Here's how the part is built. I have some questions about the finished solid (model axes, mm). A direction names the side the tool comes from. Round coordinates to 2 decimals unless told otherwise and drop trailing zeros. Write item = value, one per line. Start each with the question number.
(1) On a 3-axis mill with a long thin cutter (end or side, diameter ignored), from which of +Z, -Z, +X, -X, +Y, -Y can I reach the whole of each face in a straight line? I mean faces 4 (the cylindrical face through (95.78, -4.1, 144.76)), 5 (the cylindrical face through (127.856, -12.905, 148.568)), 6 (the flat face through (138.989, 0, 132)). Say none if no direction works.
(2) If we mould it in two halves opening along Z, with no side actions, what happens to faces 1 (the flat face through (70.307, -14, 132)), 2 (the cylindrical face through (-221.722, -170.011, -6.439)), 3 (the flat face through (0, 0, 158.217))? For each: released by +Z, released by -Z, zero draft, split by the parting line, or undercut.
(3) Will these pins go through, and if not, where does the flat tip stop? pin 1 Ø12 at (x, y) = (145, 214.5) entering from +Z; pin 2 Ø21 at (y, z) = (7.5, 141) entering from -X; pin 3 Ø1.5 at (x, z) = (123, 2) entering from +Y.
(4) I need wall thicknesses on line 1 along Z through (x, y) = (205, 138.5); line 2 along Z through (x, y) = (124.5, 5); line 3 along Y through (x, z) = (32.5, 5.5). Which ranges of each line are inside material? Lowest first, please.
```python
from build123d import *

# Parameters (mm, degrees)
EXTRUSION1_DEPTH      = 25.4
EXTRUSION1_DEPTH_BACK = 38.1
SKETCH1_R             = 279.4
FILLET1_R             = 25.4
SKETCH2_R             = 48.9585
EXTRUSION2_DEPTH      = 37.211
SKETCH3_R             = 14.9225
EXTRUSION3_DEPTH      = 95.6056
SKETCH4_R             = 13.6525
EXTRUSION4_DEPTH      = 133.8072
EXTRUSION5_START      = -80.4672
SKETCH5_R             = 21.209
SKETCH5_R_2           = 13.6525
EXTRUSION5_DEPTH      = 80.4672
EXTRUSION6_START      = -63.5
SKETCH6_R             = 21.209
EXTRUSION6_DEPTH      = 63.5
SKETCH7_R             = 13.6525
EXTRUSION7_DEPTH      = 51.6636
SKETCH8_R             = 21.209
EXTRUSION8_DEPTH      = 17.018
FILLET2_R             = 5.08


with BuildPart() as part:
    # Sketch1 → Extrusion1 (new, two sides: drawn at the far end of the back side and taken through both)
    with BuildSketch(Plane.XY.offset(-EXTRUSION1_DEPTH_BACK)):
        Circle(SKETCH1_R)
    extrude(amount=EXTRUSION1_DEPTH + EXTRUSION1_DEPTH_BACK)

    # Fillet1
    fillet1_edges = [part.edges().sort_by_distance(p)[0] for p in [
        (-279.4, 0, -38.1),
        (-279.4, 0, 25.4),
    ]]
    fillet(fillet1_edges, radius=FILLET1_R - 0.0001)  # a hair under: the kernel refuses the full size

    # Sketch2 → Extrusion2 (add)
    with BuildSketch(Plane.XY.offset(25.4)):
        with Locations(Location((0, 0, 0), (0, 0, 180))):
            Circle(SKETCH2_R)
    extrude(amount=EXTRUSION2_DEPTH)

    # Sketch3 → Extrusion3 (add)
    with BuildSketch(Plane.XY.offset(62.611)):
        Circle(SKETCH3_R)
    extrude(amount=EXTRUSION3_DEPTH)

    # Sketch4 → Extrusion4 (add)
    with BuildSketch(Plane.YZ):
        with Locations(Location((0, 131.7371, 0), (0, 0, 270))):
            Circle(SKETCH4_R)
    extrude(amount=EXTRUSION4_DEPTH)

    # Sketch5 → Extrusion5 (add)
    with BuildSketch(Plane(origin=(133.8072, 0, 0), x_dir=(0, 0, -1), z_dir=(1, 0, 0)).offset(EXTRUSION5_START)):
        with Locations((-131.7371, 0)):
            Circle(SKETCH5_R)
        with Locations(Location((-131.7371, 0, 0), (0, 0, 180))):
            Circle(SKETCH5_R_2, mode=Mode.SUBTRACT)
    extrude(amount=EXTRUSION5_DEPTH)

    # Sketch6 → Extrusion6 (cut)
    with BuildSketch(Plane(origin=(133.8072, 0, 0), x_dir=(0, 0, -1), z_dir=(1, 0, 0)).offset(EXTRUSION6_START)):
        with Locations((-131.7371, 0)):
            Circle(SKETCH6_R)
    extrude(amount=EXTRUSION6_DEPTH, mode=Mode.SUBTRACT)

    # Sketch7 → Extrusion7 (add)
    with BuildSketch(Plane(origin=(70.3072, 0, 0), x_dir=(0, 0, -1), z_dir=(1, 0, 0))):
        with Locations(Location((-131.7371, 0, 0), (0, 0, 180))):
            Circle(SKETCH7_R)
    extrude(amount=EXTRUSION7_DEPTH)

    # Sketch8 → Extrusion8 (add)
    with BuildSketch(Plane(origin=(121.9708, 0, 0), x_dir=(0, 0, -1), z_dir=(1, 0, 0))):
        with Locations((-131.7371, 0)):
            Circle(SKETCH8_R)
    extrude(amount=EXTRUSION8_DEPTH)

    # Fillet2
    fillet2_edges = [part.edges().sort_by_distance(p)[0] for p in [
        (138.9888, 0, 152.9461),
    ]]
    fillet(fillet2_edges, radius=FILLET2_R)


solid = part.part
```
Returned:
q1.face_4 = none
q1.face_5 = +X
q1.face_6 = +Z, +X, +Y, -Y
q2.face_1 = undercut
q2.face_2 = zero draft
q2.face_3 = released by +Z
q3.pin_1 = 25.4
q3.pin_2 = -14.92
q3.pin_3 = 251.15
q4.line_1 = -38.1 to 25.4
q4.line_2 = -38.1 to 25.4, 111.13 to 152.35
q4.line_3 = -276.9 to 276.9
